```python
from build123d import *

# Parameters (mm, degrees)
F1_DEPTH  = 10
F2_R      = 3
F3_DEPTH  = 10
F4_R      = 4.5
F4_R_2    = 3
F5_DEPTH  = 5
F6_R      = 4.5
F7_DEPTH  = 5
F8_DEPTH  = 5
F10_DEPTH = 14
F11_R     = 10
F12_DEPTH = 20
F13_R     = 10
F14_DEPTH = 40
F15_R     = 12
F15_R_2   = 10
F16_DEPTH = 10


with BuildPart() as f1:
    # F0 (on Front) → F1 (new body)
    with BuildSketch(Plane.XZ):
        with BuildLine():
            Line((32.1521708727, 21.1400806223), (-1.0192576987, 28.9282977823))
            ThreePointArc((-1.0192576987, 28.9282977823), (-4.4478291273, 29.3253906074), (-7.8764005559, 28.9282977823))
            Line((-7.8764005559, 28.9282977823), (-41.0478291273, 21.1400806223))
            ThreePointArc((-41.0478291273, 21.1400806223), (-46.4478291273, 14.3253906074), (-41.0478291273, 7.5107005924))
            Line((-41.0478291273, 7.5107005924), (-7.8764005559, -0.2775165675))
            ThreePointArc((-7.8764005559, -0.2775165675), (-4.4478291273, -0.6746093926), (-1.0192576987, -0.2775165675))
            Line((-1.0192576987, -0.2775165675), (32.1521708727, 7.5107005924))
            ThreePointArc((32.1521708727, 7.5107005924), (37.5521708727, 14.3253906074), (32.1521708727, 21.1400806223))
        make_face()
    extrude(amount=F1_DEPTH)

    # F2 (on face) → F3 (cut)
    with BuildSketch(Plane.XZ.offset(10)):
        with Locations((-39.4478291273, 14.3253906074)):
            Circle(F2_R)
        with Locations((30.5521708727, 14.3253906074)):
            Circle(F2_R)
    extrude(amount=-F3_DEPTH, mode=Mode.SUBTRACT)

    # F4 (on face) → F5 (join)
    with BuildSketch(Plane.XZ.offset(10)):
        with Locations((-39.4478291273, 14.3253906074)):
            Circle(F4_R)
        with Locations((-39.4478291273, 14.3253906074)):
            Circle(F4_R_2, mode=Mode.SUBTRACT)
        with Locations((30.5521708727, 14.3253906074)):
            Circle(F4_R)
        with Locations((30.5521708727, 14.3253906074)):
            Circle(F4_R_2, mode=Mode.SUBTRACT)
    extrude(amount=-F5_DEPTH)

    # F6 (on Front) → F7 (cut)
    with BuildSketch(Plane.XZ):
        with Locations((-39.4478291273, 14.3253906074)):
            Circle(F6_R)
    extrude(amount=-F7_DEPTH, mode=Mode.SUBTRACT)

    # F6 (on Front) → F8 (cut)
    with BuildSketch(Plane.XZ):
        with Locations((-39.4478291273, 14.3253906074)):
            Circle(F6_R)
        with Locations((30.5521708727, 14.3253906074)):
            Circle(F6_R)
    extrude(amount=F8_DEPTH, mode=Mode.SUBTRACT)

    # F9 (on face) → F10 (join)
    with BuildSketch(Plane(origin=(0, 0, 0), x_dir=(-1, 0, 0), z_dir=(0, 1, 0))):
        with BuildLine():
            ThreePointArc((7.8764005559, -0.2775165675), (16.2042863196, 5.0095055563), (19.4478291273, 14.3253906074))
            ThreePointArc((19.4478291273, 14.3253906074), (16.2042863196, 23.6412756585), (7.8764005559, 28.9282977823))
            ThreePointArc((7.8764005559, 28.9282977823), (4.4478291273, 29.3253906074), (1.0192576987, 28.9282977823))
            ThreePointArc((1.0192576987, 28.9282977823), (-10.5521708727, 14.3253906074), (1.0192576987, -0.2775165675))
            ThreePointArc((1.0192576987, -0.2775165675), (4.4478291273, -0.6746093926), (7.8764005559, -0.2775165675))
        make_face()
    extrude(amount=F10_DEPTH)

    # F11 (on face) → F12 (cut)
    with BuildSketch(Plane(origin=(0, 14, 0), x_dir=(-1, 0, 0), z_dir=(0, 1, 0))):
        with Locations((4.4478291273, 14.3253906074)):
            Circle(F11_R)
    extrude(amount=F12_DEPTH, mode=Mode.SUBTRACT)

    # F13 (on face) → F14 (cut)
    with BuildSketch(Plane(origin=(0, 14, 0), x_dir=(-1, 0, 0), z_dir=(0, 1, 0))):
        with Locations((4.4478291273, 14.3253906074)):
            Circle(F13_R)
    extrude(amount=-F14_DEPTH, mode=Mode.SUBTRACT)

    # F15 (on face) → F16 (cut)
    with BuildSketch(Plane(origin=(0, 14, 0), x_dir=(-1, 0, 0), z_dir=(0, 1, 0))):
        with Locations((4.4478291273, 14.3253906074)):
            Circle(F15_R)
        with Locations((4.4478291273, 14.3253906074)):
            Circle(F15_R_2, mode=Mode.SUBTRACT)
    extrude(amount=-F16_DEPTH, mode=Mode.SUBTRACT)


solid = f1.part
```
The listing builds one solid part. Answer for the finished solid, in the listing's coordinates (mm). A direction names the side the tool comes from. Round coordinates to 2 decimals unless told otherwise and drop trailing zeros. Loops run counter-clockwise (first coordinate to the right, second up) from the corner with the lowest first, then second, coordinate; pieces in that order, holes last. Notation, with made-up numbers: (51, -3) - (75, -3) arc R23 cw to (75, 16) - close; hole circle Ø4 at (26.5, -22.5). An arc over 180 degrees is marked (long way). Return JSON: item names as keys, results as strings. Group by question number.
1. The part is cut by section B-B on y = 8.25. Determine the outline of the cut face in (x, z), then the cut area to 3 significant figures.
2. The mould has two halves that part along Z. Classify faces 3 (the cylindrical face through (-38.064, -7.535, 11.664)), 4 (the cylindrical face through (-46.447, -4.93, 14.457)), 5 (the flat face through (-39, -5, 11)), 6 (the flat face through (15.8, -4.93, 24.98)): pulls with the +Z half, pulls with the -Z half, needs draft (parallel to the pull), parting line crosses it, or undercut.
3. Consider probe 1 along X at (y, z) = (11, 14.5); probe 2 along X at (y, z) = (-6.75, 11); probe 3 along Z at (x, y) = (31.5, -1). Determine where each line is inside the solid, lowest interval first.
4. Which of the six approach directions +Z, -Z, +X, -X, +Y, -Y give full straight-line access (tool end or side, diameter ignored) to faces 1 (the cylindrical face through (31.936, -7.535, 11.664)), 2 (the flat face through (-1.7, 4, 24.2))?
5. The part is cut by section C-C on z = 13.25. State how many separate pieces and enclosed holes the cut face has, then the cut area to 3 significant figures.
6. The part is cut by section D-D on x = 28.5. Determine the outline of the cut face in (y, z).
7. Each of these flat-tipped pins is pushed along its axis until it touches: P1, Ø7, axis at x = -37.5, z = 13, coming from the +Y side; P2, Ø18, axis at x = -4.45, z = 14.33, coming from the -Y side; P3, Ø2.5, axis at x = 31.5, z = 12.5, coming from the +Y side; P4, Ø1, axis at y = -7, z = 8.5, coming from the +X side. Where does it stop, or does it pass through?
8. The part is cut by section A-A on y = -1. Determine the outline of the cut face in (x, z).
Resolved:
{
 "1": {"outline": "circle Ø30 at (-4.45, 14.33); hole circle Ø24 at (-4.45, 14.33)", "area": "254 mm²"},
 "2": {"face 3": "undercut", "face 4": "parting line crosses it", "face 5": "undercut", "face 6": "pulls with the +Z half"},
 "3": {"probe 1": "x = -19.45 to -16.45, 7.55 to 10.55", "probe 2": "x = -45.61 to -13.88, 4.98 to 36.71", "probe 3": "z = 7.36 to 9.93, 18.72 to 21.29"},
 "4": {"face 1": "+Y, -Y", "face 2": "+Y"},
 "5": {"separate pieces": "4", "enclosed holes": "0", "area": "596 mm²"},
 "6": {"outline": "(-10, 6.65) - (0, 6.65) - (0, 10.32) - (-5, 10.32) - (-5, 12.14) - (-10, 12.14) - close; (-10, 16.51) - (-5, 16.51) - (-5, 18.33) - (0, 18.33) - (0, 22) - (-10, 22) - close"},
 "7": {"P1": "stops at y = 0", "P2": "passes through", "P3": "stops at y = -5", "P4": "stops at x = 35.1"},
 "8": {"outline": "(-41.05, 7.51) - (-7.88, -0.28) arc R15 ccw to (-1.02, -0.28) - (32.15, 7.51) arc R7 ccw to (32.15, 21.14) - (-1.02, 28.93) arc R15 ccw to (-7.88, 28.93) - (-41.05, 21.14) arc R7 ccw to start; hole circle Ø9 at (-39.45, 14.33); hole circle Ø20 at (-4.45, 14.33); hole circle Ø9 at (30.55, 14.33)"}
}
